```python
from build123d import *

# Parameters (mm, degrees)
SKETCH1_R           = 8.98338725
BOSS_EXTRUDE2_DEPTH = 10
CUT_EXTRUDE1_DEPTH  = 9
SKETCH9_R           = 3.37330117
CUT_EXTRUDE4_DEPTH  = 10
CUT_EXTRUDE5_DEPTH  = 10
CIRPATTERN2_COUNT   = 10
CIRPATTERN2_ANGLE   = 270


with BuildPart() as part:
    # Sketch1 → Boss-Extrude2 (new body)
    with BuildSketch(Plane.XY):
        Circle(SKETCH1_R)
    extrude(amount=-BOSS_EXTRUDE2_DEPTH)

    # Sketch2 → Cut-Extrude1 (cut)
    with BuildSketch(Plane.XY):
        with BuildLine():
            Line((-1.97475772, 2.477093755), (4.365982639, 7.851079039))
            ThreePointArc((4.365982639, 7.851079039), (6.497023817, 6.204025146), (8.044056542, 3.999300044))
            Line((8.044056542, 3.999300044), (2.911023025, -2.008935037))
            ThreePointArc((2.911023025, -2.008935037), (-2.230434429, -2.704958194), (-1.97475772, 2.477093755))
        make_face()
    extrude(amount=-CUT_EXTRUDE1_DEPTH, mode=Mode.SUBTRACT)

    # Sketch9 → Cut-Extrude4 (cut)
    with BuildSketch(Plane.XY):
        with Locations((0.051031531, -0.220189823)):
            Circle(SKETCH9_R)
    extrude(amount=-CUT_EXTRUDE4_DEPTH, mode=Mode.SUBTRACT)

    # Sketch10 → Cut-Extrude5 (cut)
    with BuildSketch(Plane.XY):
        with BuildLine():
            ThreePointArc((-0.030614018, 6.232538227), (0.505170096, 6.710825662), (0.759385982, 7.382538227))
            ThreePointArc((0.759385982, 7.382538227), (1.276411254, 8.232191257), (2.069385982, 8.832538227))
            ThreePointArc((2.069385982, 8.832538227), (-0.030614018, 8.990934274), (-2.130614018, 8.832538227))
            ThreePointArc((-2.130614018, 8.832538227), (-1.33763929, 8.232191257), (-0.820614018, 7.382538227))
            ThreePointArc((-0.820614018, 7.382538227), (-0.566398131, 6.710825662), (-0.030614018, 6.232538227))
        make_face()
    cut_extrude5 = extrude(amount=-CUT_EXTRUDE5_DEPTH, mode=Mode.SUBTRACT)

    # CirPattern2: Cut-Extrude5 ×10 about axis
    cirpattern2_axis = Axis((0, 0, 0), (0, 0, 1))
    for i in range(1, CIRPATTERN2_COUNT):
        add(cut_extrude5.rotate(cirpattern2_axis, i * CIRPATTERN2_ANGLE / (CIRPATTERN2_COUNT - 1)), mode=Mode.SUBTRACT)


solid = part.part
```
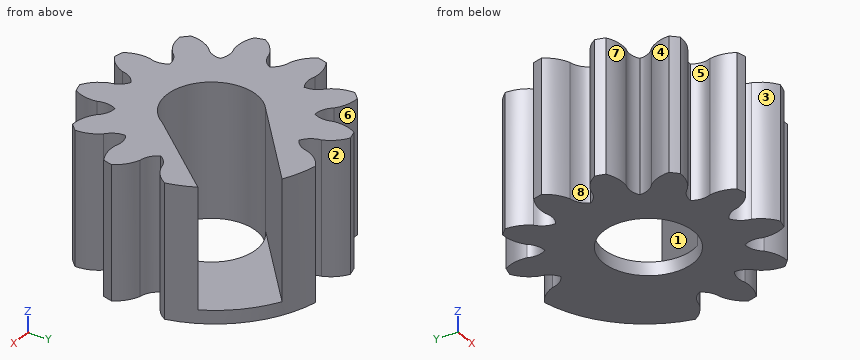
Can you work these out from the model? Positions are in its coordinate system, mm. Face numbers are marked on the shaded views. A direction names the side the tool comes from. Coordinates: 2 decimals unless noted, no trailing zeros. Loops run counter-clockwise (first coordinate to the right, second up) from the corner with the lowest first, then second, coordinate; pieces in that order, holes last. Notation, with made-up numbers: (-12.5, 68) -> (15.5, 68) arc R19 cw to (15.5, 100) -> close; hole circle Ø5 at (27.25, -37.5). An arc over 180 degrees is marked (long way). Put each result on its own line as item: value. Start each with the question number.
Q1. I want a section at C-C (y = 5). Write out the boundary of the cut face in (x, z).
Q2. I want a section at A-A (x = 0.5). Write out the boundary of the cut face in (y, z).
Q3. Thinking about a two-plate mould opening in Y: for the marked faces 6, 7 and 8, which applies, pulls with the +Y half, pulls with the -Y half, needs draft (parallel to the pull), parting line crosses it, or undercut?
Q4. I'm going to push a flat-ended pin straight in: P1, Ø5, axis at x = 5, z = -3, coming from the -Y side. Where does the tip first touch, or does it pass through?
Q5. I want a section at B-B (y = 0.25). Write out the boundary of the cut face in (x, z), plus the area to 3 significant figures.
Q6. If I drill on line 1 (Y direction, x = 6, z = -4.5); line 2 (X direction, y = 7.5, z = -7.5); line 3 (X direction, y = 7.25, z = -4.75), over which ranges is the centre line in solid material (lowest first)? Write a range as [from, to].
Q7. I want a section at D-D (x = 5). Write out the boundary of the cut face in (y, z), plus the area to 3 significant figures.
Q8. For the marked faces 1, 2, 3, 4 and 5, which set-ups out of +Z, -Z, +X, -X, +Y, -Y let a thin tool reach every point of the face, with its end or its side?
Taken from the geometry:
1. outline: (-6.41, -10) -> (7.46, -10) -> (7.46, -9) -> (1, -9) -> (1, 0) -> (-6.41, 0) -> close
2. outline: (-6.62, -10) -> (-3.56, -10) -> (-3.56, 0) -> (-6.62, 0) -> close; (3.12, -10) -> (6.7, -10) -> (6.7, 0) -> (4.57, 0) -> (4.57, -9) -> (3.12, -9) -> close
3. face 6: pulls with the +Y half
3. face 7: pulls with the -Y half
3. face 8: undercut
4. P1: stops at y = -8.63
5. outline: (-6.43, -10) -> (-3.29, -10) -> (-3.29, 0) -> (-6.43, 0) -> close; (3.39, -10) -> (6.37, -10) -> (6.37, 0) -> (4.84, 0) -> (4.84, -9) -> (3.39, -9) -> close
5. area: 48.1 mm2
6. line 1: y = [-6.59, -4.34], [-2.88, 1.61]
6. line 2: x = [-3.05, -0.87], [0.81, 3.95]
6. line 3: x = [-3.07, -0.8], [0.74, 3.66]
7. outline: (-6.35, -10) -> (7.46, -10) -> (7.46, -9) -> (0.44, -9) -> (0.44, 0) -> (-6.35, 0) -> close
7. area: 74.9 mm2
8. face 1: +Z
8. face 2: +Z, -Z, +Y
8. face 3: +Z, -Z, -Y
8. face 4: +Z, -Z, -X
8. face 5: +Z, -Z
